from build123d import *

# Parameters (mm, degrees)
CROQUIS3_R              = 7.5
SALIENTE_EXTRUIR4_DEPTH = 10


with BuildPart() as part:
    # Croquis3 → Saliente-Extruir4 (new body)
    with BuildSketch(Plane(origin=(0, 0, 0), x_dir=(1, 0, 0), z_dir=(0, 1, 0))):
        with BuildLine():
            Line((-35, -175), (35, -175))
            Line((35, -175), (35, 165))
            ThreePointArc((35, 165), (32.071067812, 172.071067812), (25, 175))
            Line((25, 175), (-25, 175))
            ThreePointArc((-25, 175), (-32.071067812, 172.071067812), (-35, 165))
            Line((-35, 165), (-35, -175))
        make_face()
        with Locations((0, 145)):
            Circle(CROQUIS3_R, mode=Mode.SUBTRACT)
        with Locations((0, 55)):
            Circle(CROQUIS3_R, mode=Mode.SUBTRACT)
        with Locations((0, -35)):
            Circle(CROQUIS3_R, mode=Mode.SUBTRACT)
    extrude(amount=SALIENTE_EXTRUIR4_DEPTH)


solid = part.part
Read the model definition and answer for the solid it produces. Units are mm, in the model's axes. Give positions to 0.01 mm unless a question says otherwise; leave off trailing zeros. Write each loop counter-clockwise with the first axis right and the second up, starting at its lowest first coordinate (ties: lowest second). Pieces come first, ordered by that corner, then holes. Notation, with made-up numbers: (-32, 57.5) -> (23, 57.5) arc R9 cw to (23, 62.5) -> close; hole circle Ø9 at (-37, 72.25). An arc over 180 degrees is marked (long way). Answer as a JSON object with one key per item and string values. Group by question number.
1) The mould has two halves that part along X. Classify faces 1 (the cylindrical face through (-31.99, 4.93, -172.15)), 2 (the cylindrical face through (-1.63, 4.93, 42.32)), 3 (the flat face through (0, 0, -2)): +X half, -X half, draft (parallel to the pull), parting line (faces both ways), or undercut.
2) Find section B-B (x = 0). Write down the section's boundary in (y, z), and give its area (3 significant figures).
3) Find section C-C (y = 6). Write down the section's boundary in (x, z), and give its area (3 significant figures).
4) Find section A-A (z = 35). Write down the section's boundary in (x, y).
5) Consider L1, parallel to Z at x = 0, y = 5.5; L2, parallel to X at y = 3.5, z = -145; L3, parallel to Z at x = -5, y = 5.5. Determine where each line is inside the solid, lowest interval first. Write a range as from..to.
Values follow:
{
 "1": {"face 1": "-X half", "face 2": "undercut", "face 3": "draft"},
 "2": {"outline": "(0, -175) -> (10, -175) -> (10, -152.5) -> (0, -152.5) -> close; (0, -137.5) -> (10, -137.5) -> (10, -62.5) -> (0, -62.5) -> close; (0, -47.5) -> (10, -47.5) -> (10, 27.5) -> (0, 27.5) -> close; (0, 42.5) -> (10, 42.5) -> (10, 175) -> (0, 175) -> close", "area": "3,050 mm2"},
 "3": {"outline": "(-35, -165) arc R10 ccw to (-25, -175) -> (25, -175) arc R10 ccw to (35, -165) -> (35, 175) -> (-35, 175) -> close; hole circle Ø15 at (0, -145); hole circle Ø15 at (0, -55); hole circle Ø15 at (0, 35)", "area": "23,900 mm2"},
 "4": {"outline": "(-35, 0) -> (-7.5, 0) -> (-7.5, 10) -> (-35, 10) -> close; (7.5, 0) -> (35, 0) -> (35, 10) -> (7.5, 10) -> close"},
 "5": {"L1": "z = -175..-152.5, -137.5..-62.5, -47.5..27.5, 42.5..175", "L2": "x = -35..-7.5, 7.5..35", "L3": "z = -175..-150.59, -139.41..-60.59, -49.41..29.41, 40.59..175"}
}
